Design review of the part built by this model. Coordinates are the model's own, in mm. A direction names the side the tool comes from. Round coordinates to 2 decimals unless told otherwise and drop trailing zeros. Order: outer loops, then holes, each group sorted by start corner. A loop starts at its lowest first (then second) coordinate and runs counter-clockwise, first axis right, second up. Notation, with made-up numbers: (-23, 84) - (21, 84) arc R23 cw to (21, 118) - close; hole circle Ø8 at (38.25, 3). An arc over 180 degrees is marked (long way). Write item = value, one per line.
from build123d import *

# Parameters (mm, degrees)
F2_R     = 7
F3_DEPTH = 20.001
F2_R_2   = 3
F4_DEPTH = 15
F2_R_3   = 9
F5_DEPTH = 3
F6_SIZE  = 0.5
F7_SIZE  = 0.5


with BuildPart() as f1:
    # F0 (on Front) → F1 (revolve)
    with BuildSketch(Plane.XZ):
        Polygon((0, -10), (0, 10), (-22.87, 10), (-22.87, 8), (-21.87, 8), (-21.87, 6.5), (-19.5, 6.5), (-19.5, 2.5), (-21.72, 2.5), (-21.72, -10), align=None)
    revolve(axis=Axis((0, 0, 0), (0, 0, -1)))

    # F2 (on face) → F3 (cut, through all)
    with BuildSketch(Plane.XY.offset(10)):
        Circle(F2_R)
    extrude(amount=-F3_DEPTH, mode=Mode.SUBTRACT)

    # F2 (on face) → F4 (cut)
    with BuildSketch(Plane.XY.offset(10)):
        with Locations((-10.960155, 10.960155)):
            Circle(F2_R_2)
        with Locations((10.960155, 10.960155)):
            Circle(F2_R_2)
        with Locations((15.5, 0)):
            Circle(F2_R_2)
        with Locations((10.960155, -10.960155)):
            Circle(F2_R_2)
        with Locations((0, -15.5)):
            Circle(F2_R_2)
        with Locations((-10.960155, -10.960155)):
            Circle(F2_R_2)
        with Locations((-15.5, 0)):
            Circle(F2_R_2)
        with Locations((0, 15.5)):
            Circle(F2_R_2)
    extrude(amount=-F4_DEPTH, mode=Mode.SUBTRACT)

    # F2 (on face) → F5 (cut)
    with BuildSketch(Plane.XY.offset(10)):
        Circle(F2_R_3)
        Circle(F2_R, mode=Mode.SUBTRACT)
    extrude(amount=-F5_DEPTH, mode=Mode.SUBTRACT)

    # F6
    f6_edges = [f1.edges().sort_by_distance(p)[0] for p in [
        (22.87, 0, 10),
        (-13.960155, -10.960155, 10),
        (-3, -15.5, 10),
        (7.960155, -10.960155, 10),
        (-18.5, 0, 10),
        (-13.960155, 10.960155, 10),
        (-9, 0, 10),
        (12.5, 0, 10),
        (-3, 15.5, 10),
        (7.960155, 10.960155, 10),
    ]]
    chamfer(f6_edges, length=F6_SIZE)

    # F7
    f7_edges = [f1.edges().sort_by_distance(p)[0] for p in [
        (22.87, 0, 8),
        (21.87, 0, 6.5),
        (21.72, 0, 2.5),
        (21.72, 0, -10),
    ]]
    chamfer(f7_edges, length=F7_SIZE)


solid = f1.part
Item 1: For line 1 along Y through (x, z) = (0, 1); line 2 along X through (y, z) = (-10, 3.75); line 3 along X through (y, z) = (13.5, 6.25), list the stretches that pass through material, from the lowest coordinate up. Write a range as [from, to].
Data:
line_1 = [-21.72, -18.5], [-12.5, -7], [7, 12.5], [18.5, 21.72]
line_2 = [-16.74, -13.8], [-8.12, 8.12], [13.8, 16.74]
line_3 = [-14.07, -12.56], [-9.36, -2.24], [2.24, 9.36], [12.56, 14.07]
Item 2: For faces 1 (the face through (-11, -11, -5)), 2 (the face through (4.958, -22.326, 8.993)), 3 (the face through (21.7, 0.95, -3.83)), list the 3-axis set-ups (+Z, -Z, +X, -X, +Y, -Y) from which the entire face can be reached by the end or side of a thin tool; tool diameter is ignored.
Data:
face_1 = +Z
face_2 = +Z, -Z
face_3 = -Z
Item 3: The part is to be moulded in two halves that separate along Z. For faces 4 (the face through (2.539, 19.334, 4.472)), 5 (the face through (-11, 11, -5)), 6 (the face through (8.579, 9.135, 2.351)), say which applies: +Z half, -Z half, draft (parallel to the pull), parting line (faces both ways), or undercut.
Data:
face_4 = undercut
face_5 = +Z half
face_6 = draft
Item 4: Take a section at A-A, the plane z = -6.25. State the section outline as (x, y) points.
Data:
outline = circle Ø43.44 at (0, 0); hole circle Ø14 at (0, 0)
Item 5: Insertion check: P1, Ø5.5, axis at x = -4, y = 4.5, coming from the +Z side; P2, Ø4, axis at x = -16, z = -3.5, coming from the -Y side; P3, Ø5, axis at x = 11.5, y = -10.5, coming from the +Z side; P4, Ø1, axis at x = -5.5, y = -2.5, coming from the +Z side. Each pin has a flat end and moves straight along its axis. Give the tip position at first contact, or say it passes through.
Data:
P1 = 7
P2 = -16.61
P3 = 9.71
P4 = through
